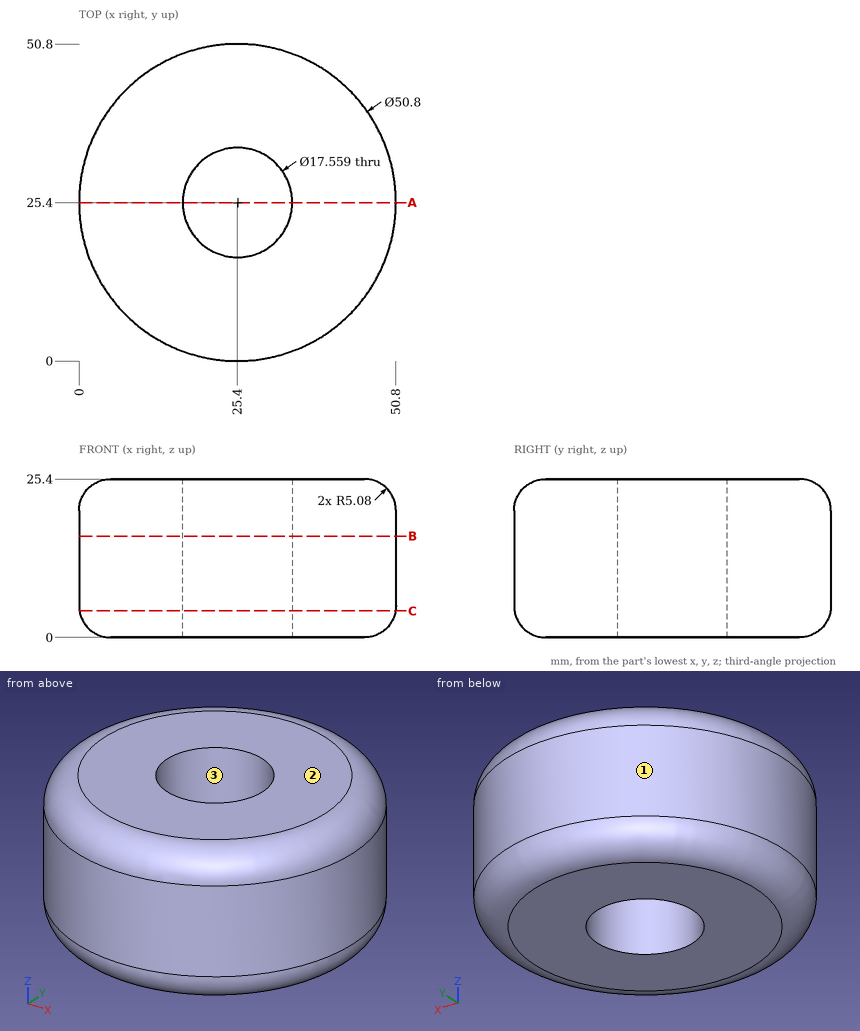
Input: dimensioned drawing with shaded views. Units: mm. Origin: part minimum x, y, z. Give positions to 0.01 mm unless a question says otherwise; leave off trailing zeros. Write each loop counter-clockwise with the first axis right and the second up, starting at its lowest first coordinate (ties: lowest second). Pieces come first, ordered by that corner, then holes. Notation, with made-up numbers: (60.25, 26) -> (112.25, 26) arc R34 ccw to (112.25, 58) -> close; hole circle Ø6 at (55.25, 74). An arc over 180 degrees is marked (long way). Answer as a JSON object with one key per item and string values.
1. Cut plane A-A on y = 25.4. Output: boundary loops of the cut face in (x, z).
Ans:
{"outline": "(0, 5.08) arc R5.08 ccw to (5.08, 0) -> (16.62, 0) -> (16.62, 25.4) -> (5.08, 25.4) arc R5.08 ccw to (0, 20.32) -> close; (34.18, 0) -> (45.72, 0) arc R5.08 ccw to (50.8, 5.08) -> (50.8, 20.32) arc R5.08 ccw to (45.72, 25.4) -> (34.18, 25.4) -> close"}
2. Ray query, probe 1 along Y at (x, z) = (25.4, 11.75); probe 2 along Y at (x, z) = (29, 5.25) (1 decimal); probe 3 along X at (y, z) = (24.5, 16.5) (1 decimal). Return the intervals inside material, ascending. Write a range as from..to.
Ans:
{"probe 1": "y = 0..16.62, 34.18..50.8", "probe 2": "y = 0.3..17.4, 33.4..50.5", "probe 3": "x = 0..16.7, 34.1..50.8"}
3. Contact query for flat-ended pins moving along their axis: pin 1 (4 mm diameter, centred on x = 45.5, z = 9.5, fed in from +Y); pin 2 (12 mm diameter, centred on y = 17, z = 16, fed in from -X); pin 3 (1 mm diameter, centred on y = 35, z = 14, fed in from -X); pin 4 (23 mm diameter, centred on x = 25.4, y = 25.4, fed in from +Z). Output: stop coordinate, or through.
Ans:
{"pin 1": "stops at y = 43.22", "pin 2": "stops at x = 0.11", "pin 3": "stops at x = 1.69", "pin 4": "stops at z = 25.4"}
4. Cut plane C-C on z = 4.25. Output: boundary loops of the cut face in (x, y), and give its area (3 significant figures).
Ans:
{"outline": "circle Ø50.66 at (25.4, 25.4); hole circle Ø17.56 at (25.4, 25.4)", "area": "1,770 mm^2"}
5. Cut plane B-B on z = 16.25. Output: boundary loops of the cut face in (x, y).
Ans:
{"outline": "circle Ø50.8 at (25.4, 25.4); hole circle Ø17.56 at (25.4, 25.4)"}
6. Mould query, pull axis X, two halves, no side actions, for the marked faces 1, 2 and 3. Classes: pulls with the +X half, pulls with the -X half, needs draft (parallel to the pull), parting line crosses it, or undercut.
Ans:
{"face 1": "parting line crosses it", "face 2": "needs draft", "face 3": "undercut"}
